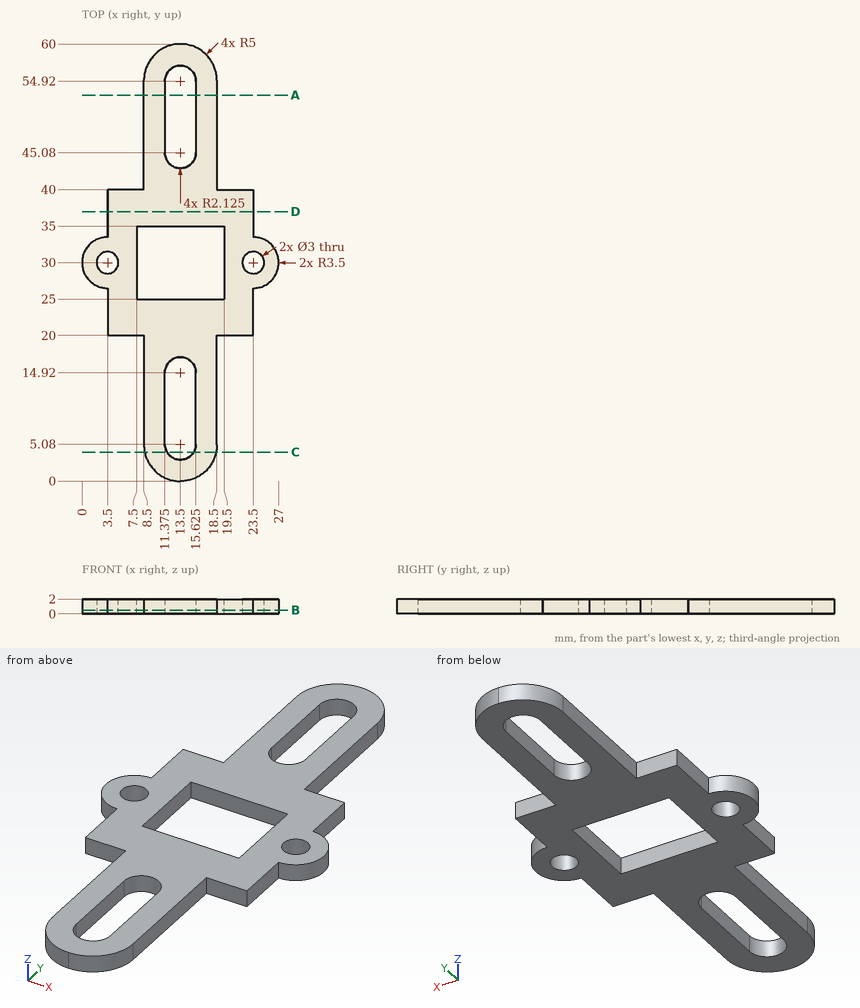
Part print with two shaded views. Sizes in mm from the minimum x, y, z corner. Coordinates: 2 decimals unless noted, no trailing zeros. Write each loop counter-clockwise with the first axis right and the second up, starting at its lowest first coordinate (ties: lowest second). Pieces come first, ordered by that corner, then holes. Notation, with made-up numbers: (61, 29) - (73, 29) arc R33 ccw to (73, 67) - close; hole circle Ø6 at (69, 58). An arc over 180 degrees is marked (long way). Put each result on its own line as item: value.
1. Flat gauge pins, fed straight in: pin 1 Ø0.6 at (x, z) = (7, 0.5) entering from -Y; pin 2 Ø0.6 at (y, z) = (36, 1.5) entering from +X; pin 3 Ø1 at (x, z) = (5, 0.5) entering from +Y. Where does each tip first touch, or does it go through?
Final values:
pin 1: stops at y = 20
pin 2: stops at x = 23.5
pin 3: stops at y = 40
2. Band-saw the part on D-D (y = 37). Write the cut outline in (x, z).
Final values:
outline: (3.5, 0) - (23.5, 0) - (23.5, 2) - (3.5, 2) - close
3. Band-saw the part on C-C (y = 4). Write the cut outline in (x, z).
Final values:
outline: (8.6, 0) - (11.67, 0) - (11.67, 2) - (8.6, 2) - close; (15.33, 0) - (18.4, 0) - (18.4, 2) - (15.33, 2) - close
4. Band-saw the part on B-B (z = 0.5). Give the number of separate pieces and of enclosed holes in the cut face, then the cut area to 3 significant figures.
Final values:
separate pieces: 1
enclosed holes: 5
area: 571 mm²
5. Probe line 1 along Y through (x, z) = (8, 0.3); line 2 along X through (y, z) = (46, 1.85) (1 decimal); line 3 along Y through (x, z) = (13, 1.8) (1 decimal). List the from-to ranges inside material, lowest first. Write a range as [from, to].
Final values:
line 1: y = [20, 25], [35, 40]
line 2: x = [8.5, 11.4], [15.6, 18.5]
line 3: y = [0, 3], [17, 25], [35, 43], [57, 60]
6. Band-saw the part on A-A (y = 53). Write the cut outline in (x, z) (1 decimal).
Final values:
outline: (8.5, 0) - (11.4, 0) - (11.4, 2) - (8.5, 2) - close; (15.6, 0) - (18.5, 0) - (18.5, 2) - (15.6, 2) - close
